from build123d import *

# Parameters (mm, degrees)
SKETCH2_W           = 184.15
SKETCH2_H           = 50.8
BOSS_EXTRUDE1_DEPTH = 1.5875
SKETCH3_R           = 1.55
CUT_EXTRUDE1_DEPTH  = 5.08


with BuildPart() as part:
    # Sketch2 → Boss-Extrude1 (new body, symmetric)
    with BuildSketch(Plane.XY):
        Rectangle(SKETCH2_W, SKETCH2_H)
    extrude(amount=BOSS_EXTRUDE1_DEPTH, both=True)

    # Sketch3 → Cut-Extrude1 (cut)
    with BuildSketch(Plane(origin=(0, 0, -1.5875), x_dir=(-1, 0, 0), z_dir=(0, 0, -1))):
        with Locations((-51.535, 8.49)):
            Circle(SKETCH3_R)
        with Locations((-64.135, -8.51)):
            Circle(SKETCH3_R)
        with Locations((64.135, 8.51)):
            Circle(SKETCH3_R)
        with Locations((51.535, -8.49)):
            Circle(SKETCH3_R)
        with BuildLine():
            Line((-46.159267508, -10.9375), (-47.390732492, -10.9375))
            ThreePointArc((-47.390732492, -10.9375), (-49.200407902, -10.187907902), (-49.95, -8.378232492))
            Line((-49.95, -8.378232492), (-49.95, 4.918232492))
            ThreePointArc((-49.95, 4.918232492), (-49.200407902, 6.727907902), (-47.390732492, 7.4775))
            Line((-47.390732492, 7.4775), (-46.159267508, 7.4775))
            ThreePointArc((-46.159267508, 7.4775), (-44.349592098, 6.727907902), (-43.6, 4.918232492))
            Line((-43.6, 4.918232492), (-43.6, -8.378232492))
            ThreePointArc((-43.6, -8.378232492), (-44.349592098, -10.187907902), (-46.159267508, -10.9375))
        make_face()
        with BuildLine():
            Line((46.419318463, -7.4775), (47.130681537, -7.4775))
            ThreePointArc((47.130681537, -7.4775), (49.124240741, -6.651740741), (49.95, -4.658181537))
            Line((49.95, -4.658181537), (49.95, 8.118181537))
            ThreePointArc((49.95, 8.118181537), (49.124240741, 10.111740741), (47.130681537, 10.9375))
            Line((47.130681537, 10.9375), (46.419318463, 10.9375))
            ThreePointArc((46.419318463, 10.9375), (44.425759259, 10.111740741), (43.6, 8.118181537))
            Line((43.6, 8.118181537), (43.6, -4.658181537))
            ThreePointArc((43.6, -4.658181537), (44.425759259, -6.651740741), (46.419318463, -7.4775))
        make_face()
    extrude(amount=-CUT_EXTRUDE1_DEPTH, mode=Mode.SUBTRACT)


solid = part.part
Read the model definition and answer for the solid it produces. Units are mm, in the model's axes. A direction names the side the tool comes from. Give positions to 0.01 mm unless a question says otherwise; leave off trailing zeros. Answer in a Markdown table with one row per item. Add a question column.
Item 1: A tool of negligible diameter and unlimited length cuts with its end or side. For faces 4 (the face through (-49.95, 2, 0)), 5 (the face through (-1, 25.4, 0)), from which of +Z, -Z, +X, -X, +Y, -Y can it reach the whole face along a straight path? Write none if from no direction.
Item 2: Section A-A, the plane y = 0.5 is taken. Count the separate pieces of the cut face and the enclosed holes in it, and give its area (3 significant figures).
Item 3: Find the intervals of material crossed by L1, parallel to X at y = 3, z = -1.3 (3 decimals); L2, parallel to Y at x = -47.5, z = -0.7; L3, parallel to X at y = 9, z = -0.8 (3 decimals), in increasing order.
Item 4: Determine the mould class of faces 1 (the face through (92.075, 0, 0)), 2 (the face through (-1, 0, 1.588)), 3 (the face through (-1, 0, -1.588)) for opening direction Z: pulls with the +Z half, pulls with the -Z half, needs draft (parallel to the pull), parting line crosses it, or undercut.
Recorded:
| question | item | result |
|---|---|---|
| 1 | face 4 | +Z, -Z |
| 1 | face 5 | +Z, -Z, +X, -X, +Y |
| 2 | separate pieces | 3 |
| 2 | enclosed holes | 0 |
| 2 | area | 544 mm2 |
| 3 | L1 | x = -92.075 to -49.95, -43.6 to 43.6, 49.95 to 92.075 |
| 3 | L2 | y = -25.4 to -7.45, 10.91 to 25.4 |
| 3 | L3 | x = -92.075 to -65.606, -62.664 to -49.809, -43.741 to 50.071, 52.999 to 92.075 |
| 4 | face 1 | needs draft |
| 4 | face 2 | pulls with the +Z half |
| 4 | face 3 | pulls with the -Z half |
